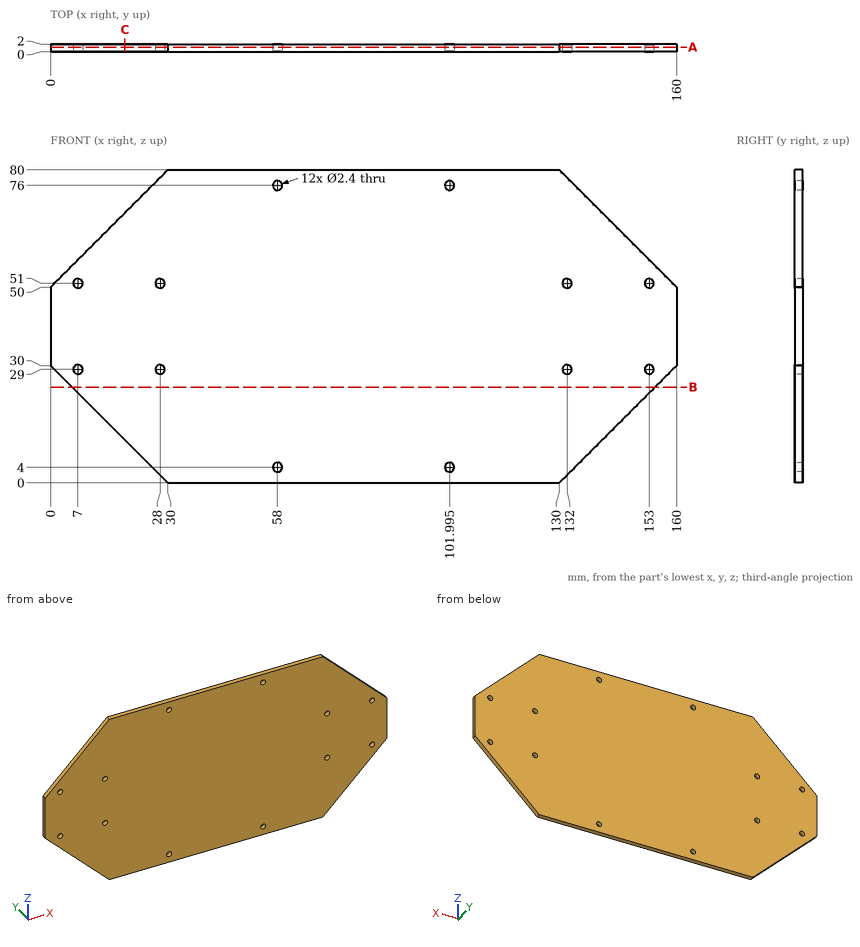
Could you check a few things on this drawing? It's one solid part, dimensions in mm from its lowest x, y, z. Round coordinates to 2 decimals unless told otherwise and drop trailing zeros. Order: outer loops, then holes, each group sorted by start corner. A loop starts at its lowest first (then second) coordinate and runs counter-clockwise, first axis right, second up. Notation, with made-up numbers: M 82,56 L 140,56 A17 cw 140,88 Z; hole C 18.25,45 d3. An arc over 180 degrees is marked long. Use a Markdown table: item, result.
1) I'm going to push a flat-ended pin straight in: P1, Ø1.9, axis at x = 101.99, z = 76, coming from the +Y side. Where does the tip first touch, or does it pass through?
Geometry says:
| item | result |
|---|---|
| P1 | passes through |
2) Imagine slicing it at C-C (x = 19). List the corners of the cut face in (y, z) for me.
Geometry says:
| item | result |
|---|---|
| outline | M 0,11 L 2,11 L 2,69 L 0,69 Z |
3) Imagine slicing it at B-B (z = 24.5). List the corners of the cut face in (x, y) for me, then the cut area to 3 significant figures.
Geometry says:
| item | result |
|---|---|
| outline | M 5.5,0 L 154.5,0 L 154.5,2 L 5.5,2 Z |
| area | 298 mm² |
4) Imagine slicing it at A-A (y = 1.2). Give the number of separate pieces and of enclosed holes in the cut face, then the cut area to 3 significant figures.
Geometry says:
| item | result |
|---|---|
| separate pieces | 1 |
| enclosed holes | 12 |
| area | 10,900 mm² |
5) If I drill on line 1 along Z through (x, y) = (58, 0.75); line 2 along X through (y, z) = (1.5, 29); line 3 along Z through (x, y) = (7, 0.75), over which ranges is the centre line in solid material (lowest first)?
Geometry says:
| item | result |
|---|---|
| line 1 | z = 0 to 2.8, 5.2 to 74.8, 77.2 to 80 |
| line 2 | x = 1 to 5.8, 8.2 to 26.8, 29.2 to 130.8, 133.2 to 151.8, 154.2 to 159 |
| line 3 | z = 23 to 27.8, 30.2 to 49.8, 52.2 to 57 |
